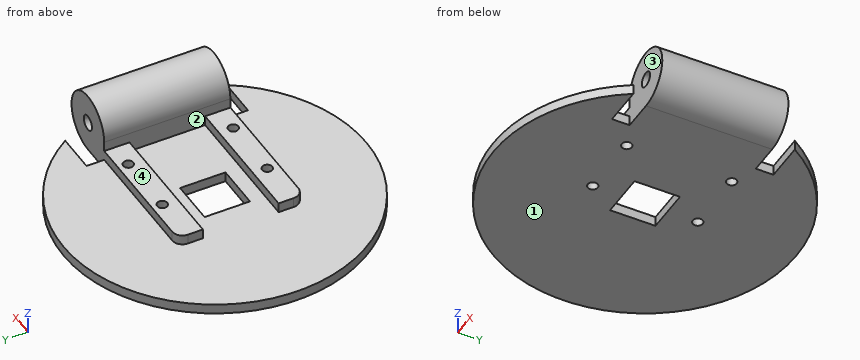
```python
from build123d import *

# Parameters (mm, degrees)
F0_R     = 1.5
F1_DEPTH = 12.5
F2_R     = 2
F3_R     = 1
F3_W     = 9
F3_H     = 9
F4_DEPTH = 2
F5_R     = 1
F6_DEPTH = 2
F8_DEPTH = 2


with BuildPart() as f1:
    # F0 (on Front) → F1 (new body, symmetric)
    with BuildSketch(Plane.XZ):
        with BuildLine():
            ThreePointArc((0, -6), (4.2426406871, 4.2426406871), (-6, 0))
            Line((-6, 0), (-6, -4))
            Line((-6, -4), (-33, -4))
            Line((-33, -4), (-33, -6))
            Line((-33, -6), (0, -6))
        make_face()
        Circle(F0_R, mode=Mode.SUBTRACT)
    extrude(amount=F1_DEPTH, both=True)

    # F2
    f2_edges = [f1.edges().sort_by_distance(p)[0] for p in [
        (-33, -12.5, -5),
        (-33, 12.5, -5),
    ]]
    fillet(f2_edges, radius=F2_R)

    # F3 (on face) → F4 (cut, through all)
    with BuildSketch(Plane.XY.offset(-4)):
        with Locations((-23.638, 10.5)):
            Circle(F3_R)
        with Locations((-11.138, 10.5)):
            Circle(F3_R)
        with Locations((-11.138, -10.3)):
            Circle(F3_R)
        with Locations((-23.638, -10.3)):
            Circle(F3_R)
        with Locations((-23.538, 0)):
            Rectangle(F3_W, F3_H)
    extrude(amount=-F4_DEPTH, mode=Mode.SUBTRACT)

    # F5 (on face) → F6 (join)
    with BuildSketch(Plane.XY.offset(-4)):
        with BuildLine():
            Line((-6, -12.5), (-6, -7.5))
            Line((-6, -7.5), (-33, -7.5))
            Line((-33, -7.5), (-33, -10.5))
            ThreePointArc((-33, -10.5), (-32.4142135624, -11.9142135624), (-31, -12.5))
            Line((-31, -12.5), (-6, -12.5))
        make_face()
        with Locations((-23.638, -10.3)):
            Circle(F5_R, mode=Mode.SUBTRACT)
        with Locations((-11.138, -10.3)):
            Circle(F5_R, mode=Mode.SUBTRACT)
        with BuildLine():
            Line((-33, 7.5), (-6, 7.5))
            Line((-6, 7.5), (-6, 12.5))
            Line((-6, 12.5), (-31, 12.5))
            ThreePointArc((-31, 12.5), (-32.4142135624, 11.9142135624), (-33, 10.5))
            Line((-33, 10.5), (-33, 7.5))
        make_face()
        with Locations((-23.638, 10.5)):
            Circle(F5_R, mode=Mode.SUBTRACT)
        with Locations((-11.138, 10.5)):
            Circle(F5_R, mode=Mode.SUBTRACT)
    extrude(amount=F6_DEPTH)

    # F7 (on face) → F8 (join, through all)
    with BuildSketch(Plane(origin=(0, 0, -6), x_dir=(1, 0, 0), z_dir=(0, 0, -1))):
        with BuildLine():
            Line((-6, 16), (1.8391550809, 16))
            ThreePointArc((1.8391550809, 16), (-53.538, 0), (1.8391550809, -16))
            Line((1.8391550809, -16), (-6, -16))
            Line((-6, -16), (-6, -12.5))
            Line((-6, -12.5), (-31, -12.5))
            ThreePointArc((-31, -12.5), (-32.4142135624, -11.9142135624), (-33, -10.5))
            Line((-33, -10.5), (-33, 10.5))
            ThreePointArc((-33, 10.5), (-32.4142135624, 11.9142135624), (-31, 12.5))
            Line((-31, 12.5), (-6, 12.5))
            Line((-6, 12.5), (-6, 16))
        make_face()
    extrude(amount=-F8_DEPTH)


solid = f1.part
```
For this review, take the finished solid that the model builds, in its own axes (mm). Face numbers are marked on the shaded views. A direction names the side the tool comes from. Give positions to 0.01 mm unless a question says otherwise; leave off trailing zeros. Write each loop counter-clockwise with the first axis right and the second up, starting at its lowest first coordinate (ties: lowest second). Pieces come first, ordered by that corner, then holes. Notation, with made-up numbers: M 5,-4.75 L 62,-4.75 A22 cw 62,29.25 Z; hole C 59.5,2 d6. An arc over 180 degrees is marked long. Answer as CSV lines item,"result".
1. For pin 1 (6 mm diameter, centred on x = -17.5, y = 16.5, fed in from +Z); pin 2 (1 mm diameter, centred on y = 13.5, z = -5, fed in from +X); pin 3 (2 mm diameter, centred on x = -2, z = -5, fed in from -Y), all flat-tipped, find the tip position at first contact; note any pin that passes through.
Findings:
pin 1,"stops at z = -4"
pin 2,"stops at x = -6"
pin 3,"stops at y = -21.87"
2. Wall thickness on line 1 (Y direction, x = -28, z = -2.5); line 2 (Z direction, x = -42, y = 13.5); line 3 (Y direction, x = 3, z = 3.5): over which ranges is each line inside the solid? List them lowest first.
Findings:
line 1,"y = -12.5 to -7.5, 7.5 to 12.5"
line 2,"z = -6 to -4"
line 3,"y = -12.5 to 12.5"
3. Draft analysis for pull direction Y (two halves, no side actions). For the marked faces 1 and 2, state which applies: +Y half, -Y half, draft (parallel to the pull), parting line (faces both ways), or undercut.
Findings:
face 1,"draft"
face 2,"undercut"
4. Consider section B-B, the plane z = 4.75. Write out the cut boundary in (x, y).
Findings:
outline,"M -3.67,-12.5 L 3.67,-12.5 L 3.67,12.5 L -3.67,12.5 Z"
5. For the marked faces 3 and 4, list the 3-axis set-ups (+Z, -Z, +X, -X, +Y, -Y) from which the entire face can be reached by the end or side of a thin tool; tool diameter is ignored.
Findings:
face 3,"+Z, +X"
face 4,"+Z, -X, +Y, -Y"
6. Consider section A-A, the plane y = 0. Write out the cut boundary in (x, z).
Findings:
outline,"M -53.54,-6 L -28.04,-6 L -28.04,-4 L -53.54,-4 Z; M -19.04,-6 L 0,-6 A6 ccw long -6,0 L -6,-4 L -19.04,-4 Z; hole C 0,0 d3"
7. Consider section C-C, the plane y = 20.5. Write out the cut boundary in (x, z).
Findings:
outline,"M -45.44,-6 L -1.63,-6 L -1.63,-4 L -45.44,-4 Z"
